Source: CAD feature listing. Evaluate the final solid. Frame: model axes, mm. A direction names the side the tool comes from. Give positions to 0.01 mm unless a question says otherwise; leave off trailing zeros. Loops run counter-clockwise (first coordinate to the right, second up) from the corner with the lowest first, then second, coordinate; pieces in that order, holes last. Notation, with made-up numbers: (-4.5, 13.5) -> (7.5, 13.5) arc R24 ccw to (7.5, 45.5) -> close; hole circle Ø8 at (-29, -8.75). An arc over 180 degrees is marked (long way). Put each result on its own line as item: value.
```python
from build123d import *

# Parameters (mm, degrees)
F1_DEPTH      = 50.8
F1_DEPTH_BACK = 50.8
F2_DEPTH      = 101.601
F1_FACE1_W    = 101.6
F1_FACE1_H    = 25.4


with BuildPart() as f1:
    # F0 (on Front) → F1 (new body, two sides)
    with BuildSketch(Plane.XZ) as f1_sk:
        Polygon((0, 25.4), (0, 0), (50.8, 0), (25.4, 25.4), align=None)
    extrude(amount=F1_DEPTH)
    extrude(f1_sk.sketch, amount=-F1_DEPTH_BACK)

    # F6 (on face) → F2 (cut, through all)
    with BuildSketch(Plane.XZ.offset(50.8)):
        with BuildLine():
            Line((0, 25.4), (25.4, 25.4))
            ThreePointArc((25.4, 25.4), (12.7, 38.1), (0, 25.4))
        make_face()
        with BuildLine():
            ThreePointArc((0, 25.4), (12.7, 12.7), (25.4, 25.4))
            Line((25.4, 25.4), (0, 25.4))
        make_face()
    extrude(amount=-F2_DEPTH, mode=Mode.SUBTRACT)

    # F4: sweep along a path in F3
    with BuildLine(Plane.XZ) as f4_path:
        ThreePointArc((36.278456417, 35.56), (-28.4094161115, 65.2691159795), (0, 0))
    # F1_face1 (on face) → F4 (sweep)
    with BuildSketch(Plane(origin=(0, 0, 12.7), x_dir=(0, -1, 0), z_dir=(-1, 0, 0))):
        Rectangle(F1_FACE1_W, F1_FACE1_H)
    sweep(path=f4_path.line)


solid = f1.part
```
(1) Line query: probe 1 along X at (y, z) = (-45, 19); probe 2 along Z at (x, y) = (23, -1); probe 3 along X at (y, z) = (-39, 20.5). Output: solid intervals per line, ascending. Write a range as from..to.
Calculated:
probe 1: x = -34.73..1.73, 23.67..31.8
probe 2: z = 0..17.97, 37.04..67.04
probe 3: x = -35.55..0.98, 24.42..30.3
(2) Section B-B on x = 12.7. Return loops of the section in (y, z).
Calculated:
outline: (-50.8, 0) -> (50.8, 0) -> (50.8, 12.7) -> (-50.8, 12.7) -> close; (-50.8, 38.2) -> (50.8, 38.2) -> (50.8, 73.32) -> (-50.8, 73.32) -> close
(3) Section A-A on z = 14.5. Return loops of the section in (x, y), then the cut area to 3 significant figures.
Calculated:
outline: (-31.68, -50.8) -> (6.18, -50.8) -> (6.18, 50.8) -> (-31.68, 50.8) -> close; (19.22, -50.8) -> (36.3, -50.8) -> (36.3, 50.8) -> (19.22, 50.8) -> close
area: 5,580 mm²
(4) Section C-C on y = -16. Return loops of the section in (x, z).
Calculated:
outline: (0, 0) -> (50.8, 0) -> (25.4, 25.4) arc R12.7 cw to (0, 25.4) arc R12.78 cw (long way) to (11.04, 38.38) -> (36.28, 35.56) arc R38.1 ccw (long way) to start
(5) Draft query along X for faces 3 (the flat face through (-11, -50.8, 25)), 4 (the cylindrical face through (-27.48, -0.71, 66.15)), 5 (the cylindrical face through (12.421, -0.711, 12.703)), 6 (the flat face through (23.83, 0.71, 36.95)). Return one class per face: released by +X, released by -X, zero draft, split by the parting line, or undercut.
Calculated:
face 3: zero draft
face 4: split by the parting line
face 5: undercut
face 6: undercut
(6) Reachability of faces 1 (the flat face through (38.3, -0.7, 12.5)), 2 (the flat face through (-15, 50.8, 40)) from +Z, -Z, +X, -X, +Y, -Y: full face, straight path, thin tool, end or side. Return the list, or none.
Calculated:
face 1: +X, +Y, -Y
face 2: +Z, -Z, +X, -X, +Y
(7) Section D-D on z = 68. Return loops of the section in (x, y).
Calculated:
outline: (-25.3, -50.8) -> (21.82, -50.8) -> (21.82, 50.8) -> (-25.3, 50.8) -> close
(8) First-contact query: P1, Ø1.5, axis at y = 5, z = 27.5, coming from the -X side; P2, Ø1.5, axis at x = 12, y = 3.5, coming from the -Z side; P3, Ø2, axis at y = -19.5, z = 18.5, coming from the -X side. Flat tips, straight axial feed; report the tip coordinate or a pass-through.
Calculated:
P1: stops at x = -38.55
P2: stops at z = 0
P3: stops at x = -35.01
